```python
from build123d import *

# Parameters (mm, degrees)
SKETCH_W     = 40
SKETCH_H     = 60
PAD_DEPTH    = 1.5
SKETCH001_R  = 1
POCKET_DEPTH = 1.501
SKETCH002_W  = 33
SKETCH002_H  = 52
PAD001_DEPTH = 21


with BuildPart() as part:
    # Sketch → Pad (new body)
    with BuildSketch(Plane.XY):
        Rectangle(SKETCH_W, SKETCH_H)
    extrude(amount=PAD_DEPTH)

    # Sketch001 (on Face6 of Pad) → Pocket (cut, through all)
    with BuildSketch(Plane.XY.offset(1.5)):
        with Locations((-18, 28)):
            Circle(SKETCH001_R)
        with Locations((18, 28)):
            Circle(SKETCH001_R)
        with Locations((-18, -28)):
            Circle(SKETCH001_R)
        with Locations((18, -28)):
            Circle(SKETCH001_R)
    extrude(amount=-POCKET_DEPTH, mode=Mode.SUBTRACT)

    # Sketch002 (on Face5 of Pocket) → Pad001 (join)
    with BuildSketch(Plane.XY.offset(1.5)):
        Rectangle(SKETCH002_W, SKETCH002_H)
    extrude(amount=PAD001_DEPTH)


solid = part.part
```
Check sheet for the modelled part. Datum: model origin and axes. Units: mm. A direction names the side the tool comes from. Round coordinates to 2 decimals unless told otherwise and drop trailing zeros. Write each loop counter-clockwise with the first axis right and the second up, starting at its lowest first coordinate (ties: lowest second). Pieces come first, ordered by that corner, then holes. Notation, with made-up numbers: (31.5, -4.75) -> (35.5, -4.75) arc R9 ccw to (35.5, 7.25) -> close; hole circle Ø8 at (-34.75, 23). An arc over 180 degrees is marked (long way). One line per question, with ' | ' between items. Start each with the question number.
1. Depth check by flat-ended pin: pin 1 (8 mm diameter, centred on y = 15.5, z = 7.5, fed in from +X); pin 2 (10.5 mm diameter, centred on x = -3, z = 15.5, fed in from -Y); pin 3 (1.6 mm diameter, centred on x = 18, y = 28, fed in from +Z); pin 4 (12 mm diameter, centred on y = -21, z = 16, fed in from -X). Enter the tip coordinate at first touch or a pass-through.
2. Scan lines: line 1 along Y through (x, z) = (18, 0.55); line 2 along X through (y, z) = (5.5, 4); line 3 along Z through (x, y) = (-1, 27). Record each from-to range of solid material in increasing order. Write a range as from..to.
3. Sectioned sample at B-B, the plane y = -28. Record the cut outline in (x, z), then the cut area to 3 significant figures.
4. Set-up check for faces 4 (the face through (16.5, 0, 12)), 5 (the face through (0, 26, 12)), 6 (the face through (-16.5, 0, 12)): record each of +Z, -Z, +X, -X, +Y, -Y from which the full face is reachable in a straight line by a thin tool's end or side.
5. Sectioned sample at C-C, the plane x = 0. Record the cut outline in (y, z).
6. Release check for a two-part mould opening along Y. For faces 1 (the face through (0, 0, 22.5)), 2 (the face through (18, 29, 1)), 3 (the face through (0, -26, 12)) record: +Y half, -Y half, draft (parallel to the pull), parting line (faces both ways), or undercut.
7. Sectioned sample at D-D, the plane z = 10. Record the cut outline in (x, y).
8. Sectioned sample at A-A, the plane x = -18. Record the cut outline in (y, z).
Taken from the geometry:
1) pin 1: stops at x = 16.5 | pin 2: stops at y = -26 | pin 3: passes through | pin 4: stops at x = -16.5
2) line 1: y = -30..-29, -27..27, 29..30 | line 2: x = -16.5..16.5 | line 3: z = 0..1.5
3) outline: (-20, 0) -> (-19, 0) -> (-19, 1.5) -> (-20, 1.5) -> close; (-17, 0) -> (17, 0) -> (17, 1.5) -> (-17, 1.5) -> close; (19, 0) -> (20, 0) -> (20, 1.5) -> (19, 1.5) -> close | area: 54.0 mm^2
4) face 4: +Z, +X, +Y, -Y | face 5: +Z, +X, -X, +Y | face 6: +Z, -X, +Y, -Y
5) outline: (-30, 0) -> (30, 0) -> (30, 1.5) -> (26, 1.5) -> (26, 22.5) -> (-26, 22.5) -> (-26, 1.5) -> (-30, 1.5) -> close
6) face 1: draft | face 2: undercut | face 3: -Y half
7) outline: (-16.5, -26) -> (16.5, -26) -> (16.5, 26) -> (-16.5, 26) -> close
8) outline: (-30, 0) -> (-29, 0) -> (-29, 1.5) -> (-30, 1.5) -> close; (-27, 0) -> (27, 0) -> (27, 1.5) -> (-27, 1.5) -> close; (29, 0) -> (30, 0) -> (30, 1.5) -> (29, 1.5) -> close
